Source: CAD feature listing. Evaluate the final solid. Frame: model axes, mm. Give positions to 0.01 mm unless a question says otherwise; leave off trailing zeros. Loops run counter-clockwise (first coordinate to the right, second up) from the corner with the lowest first, then second, coordinate; pieces in that order, holes last. Notation, with made-up numbers: (15.5, -23.5) -> (39.5, -23.5) arc R16 cw to (39.5, -17.5) -> close; hole circle Ø4 at (-2, -14). An arc over 180 degrees is marked (long way). Return JSON: item names as keys, results as strings. Group by question number.
(1) Pin query (flat end, axial travel): pin 1 (3 mm diameter, centred on x = 6, y = 0, fed in from +Z); pin 2 (0.5 mm diameter, centred on x = 8, y = 0, fed in from +Z). Return the tip coordinate at first contact, or that it passes through.
(2) Draft query along X for faces 1 (the face through (-4.984, -0.421, 0.913)), 2 (the face through (-10, 0, 1)), 3 (the face through (0, -2.75, 1)). Return one class per face: released by +X, released by -X, zero draft, split by the parting line, or undercut.
(3) Cut plane B-B on y = 0. Return loops of the section in (x, z).
(4) Cut plane C-C on x = 6. Return loops of the section in (y, z).
(5) Ray query, line 1 (Y direction, x = 6, z = 0.6); line 2 (X direction, y = -0.55, z = 2.3); line 3 (X direction, y = -0.8, z = 2.5). Return the intervals inside material, ascending. Write a range as from..to.
(6) Cut plane A-A on z = 1.4. Return loops of the section in (x, y).
(7) Cut plane D-D on z = 2.65. Return loops of the section in (x, y).
```python
from build123d import *

# Parameters (mm, degrees)
SKETCH_W        = 10
SKETCH_H        = 5.5
PAD_DEPTH       = 3
SKETCH001_R     = 1.1
POCKET_DEPTH    = 3.001
SKETCH002_W     = 0.6
SKETCH002_H     = 0.6
POCKET001_DEPTH = 5.501
FILLET_R        = 0.75
CHAMFER_SIZE    = 1.2


with BuildPart() as part:
    # Sketch → Pad (new body)
    with BuildSketch(Plane.XY):
        with Locations((-5, 0)):
            Rectangle(SKETCH_W, SKETCH_H)
    extrude(amount=PAD_DEPTH)

    # Sketch001 (on Face6 of Pad) → Pocket (cut, through all)
    with BuildSketch(Plane.XY.offset(3)):
        with Locations((-6, 0)):
            Circle(SKETCH001_R)
    extrude(amount=-POCKET_DEPTH, mode=Mode.SUBTRACT)

    # Sketch002 (on Face1 of Pocket) → Pocket001 (cut, through all)
    with BuildSketch(Plane.XZ.offset(2.75)):
        with Locations((-8, 1.5)):
            Rectangle(SKETCH002_W, SKETCH002_H)
    extrude(amount=-POCKET001_DEPTH, mode=Mode.SUBTRACT)

    # Fillet
    fillet_edges = [part.edges().sort_by_distance(p)[0] for p in [
        (-10, -2.75, 1.5),
        (-10, 2.75, 1.5),
    ]]
    fillet(fillet_edges, radius=FILLET_R)

    # Mirrored: part across YZ


with BuildPart() as part_1:
    add(part.part)
    add(part.part.mirror(Plane.YZ))

    # Chamfer
    chamfer_edges = [part_1.edges().sort_by_distance(p)[0] for p in [
        (-7.1, 0, 3),
        (7.1, 0, 3),
    ]]
    chamfer(chamfer_edges, length=CHAMFER_SIZE)


solid = part_1.part
```
Answers:
{
 "1": {"pin 1": "z = 2.2", "pin 2": "z = 2.95"},
 "2": {"face 1": "undercut", "face 2": "released by -X", "face 3": "zero draft"},
 "3": {"outline": "(-10, 0) -> (-7.1, 0) -> (-7.1, 1.8) -> (-8.3, 3) -> (-10, 3) -> close; (-4.9, 0) -> (4.9, 0) -> (4.9, 1.8) -> (3.7, 3) -> (-3.7, 3) -> (-4.9, 1.8) -> close; (7.1, 0) -> (10, 0) -> (10, 3) -> (8.3, 3) -> (7.1, 1.8) -> close; hole (-8.3, 1.2) -> (-7.7, 1.2) -> (-7.7, 1.8) -> (-8.3, 1.8) -> close; hole (7.7, 1.2) -> (8.3, 1.2) -> (8.3, 1.8) -> (7.7, 1.8) -> close"},
 "4": {"outline": "(-2.75, 0) -> (-1.1, 0) -> (-1.1, 1.8) -> (-2.3, 3) -> (-2.75, 3) -> close; (1.1, 0) -> (2.75, 0) -> (2.75, 3) -> (2.3, 3) -> (1.1, 1.8) -> close"},
 "5": {"line 1": "-2.75..-1.1, 1.1..2.75", "line 2": "-10..-7.5, -4.5..4.5, 7.5..10", "line 3": "-10..-7.61, -4.39..4.39, 7.61..10"},
 "6": {"outline": "(-10, -2) arc R0.75 ccw to (-9.25, -2.75) -> (-8.3, -2.75) -> (-8.3, 2.75) -> (-9.25, 2.75) arc R0.75 ccw to (-10, 2) -> close; (-7.7, -2.75) -> (7.7, -2.75) -> (7.7, 2.75) -> (-7.7, 2.75) -> close; (8.3, -2.75) -> (9.25, -2.75) arc R0.75 ccw to (10, -2) -> (10, 2) arc R0.75 ccw to (9.25, 2.75) -> (8.3, 2.75) -> close; hole circle Ø2.2 at (-6, 0); hole circle Ø2.2 at (6, 0)"},
 "7": {"outline": "(-10, -2) arc R0.75 ccw to (-9.25, -2.75) -> (9.25, -2.75) arc R0.75 ccw to (10, -2) -> (10, 2) arc R0.75 ccw to (9.25, 2.75) -> (-9.25, 2.75) arc R0.75 ccw to (-10, 2) -> close; hole circle Ø3.9 at (-6, 0); hole circle Ø3.9 at (6, 0)"}
}
